Build history of the part. All positions in model axes, mm. Round coordinates to 2 decimals unless told otherwise and drop trailing zeros. Loops run counter-clockwise (first coordinate to the right, second up) from the corner with the lowest first, then second, coordinate; pieces in that order, holes last. Notation, with made-up numbers: (-12.5, -22.75) -> (32.5, -22.75) arc R30 cw to (32.5, 8.25) -> close; hole circle Ø7 at (-26, -27). An arc over 180 degrees is marked (long way). Put each result on its own line as item: value. Start each with the question number.
Item 1: Pull direction X, two halves, no side cores. Call faces 1 (the cylindrical face through (125.551, -62.682, 1.528)), 2 (the cylindrical face through (1.449, -62.682, 1.528)), 3 (the cylindrical face through (63.659, -64.318, 58.462)), 4 (the cylindrical face through (64.318, -125.551, 1.528)): +X half, -X half, draft (parallel to the pull), parting line (faces both ways), or undercut.
Item 2: Cut at A-A, the plane y = -115.5. List the corners of the cut face in (x, z).
Item 3: Drill centre lines: probe 1 along X at (y, z) = (-16, 63.5); probe 2 along Z at (x, y) = (60.5, -76); probe 3 along Z at (x, y) = (54, -58.5). Where is each one in solid material? Low to high. Write a range as [from, to].
```python
from build123d import *

# Parameters (mm, degrees)
F0_W     = 127
F0_H     = 127
F1_DEPTH = 127
F2_R     = 5.08
F3_R     = 12.617279
F4_DEPTH = 127.001
F5_R     = 5.08


with BuildPart() as f1:
    # F0 (on Top) → F1 (new body)
    with BuildSketch(Plane.XY):
        with Locations((63.5, -63.5)):
            Rectangle(F0_W, F0_H)
    extrude(amount=F1_DEPTH)

    # F2
    f2_edges = [f1.edges().sort_by_distance(p)[0] for p in [
        (63.5, -127, 127),
        (127, -63.5, 127),
        (0, -63.5, 127),
        (63.5, 0, 127),
        (127, -127, 63.5),
        (63.5, -127, 0),
        (127, -63.5, 0),
        (127, 0, 63.5),
        (63.5, 0, 0),
        (0, 0, 63.5),
        (0, -63.5, 0),
        (0, -127, 63.5),
    ]]
    fillet(f2_edges, radius=F2_R)

    # F3 (on face) → F4 (cut, through all)
    with BuildSketch(Plane.XZ.offset(127)):
        with Locations((57.836652, 69.655485)):
            Circle(F3_R)
    extrude(amount=-F4_DEPTH, mode=Mode.SUBTRACT)

    # F5
    f5_edges = [f1.edges().sort_by_distance(p)[0] for p in [
        (45.219373, -127, 69.655485),
        (45.219373, 0, 69.655485),
    ]]
    fillet(f5_edges, radius=F5_R)


solid = f1.part
```
Reply:
1. face 1: +X half
1. face 2: -X half
1. face 3: undercut
1. face 4: draft
2. outline: (0, 5.08) arc R5.08 ccw to (5.08, 0) -> (121.92, 0) arc R5.08 ccw to (127, 5.08) -> (127, 121.92) arc R5.08 ccw to (121.92, 127) -> (5.08, 127) arc R5.08 ccw to (0, 121.92) -> close; hole circle Ø25.23 at (57.84, 69.66)
3. probe 1: x = [0, 46.82], [68.85, 127]
3. probe 2: z = [0, 57.32], [81.99, 127]
3. probe 3: z = [0, 57.64], [81.68, 127]
